For this review, take the finished solid that the model builds, in its own axes (mm). Give positions to 0.01 mm unless a question says otherwise; leave off trailing zeros. Loops run counter-clockwise (first coordinate to the right, second up) from the corner with the lowest first, then second, coordinate; pieces in that order, holes last.
```python
from build123d import *

# Parameters (mm, degrees)
SKETCH1_W                 = 220
SKETCH1_H                 = 220
BOSS_EXTRUDE1_DEPTH       = 6
SKETCH2_R                 = 6
CUT_EXTRUDE1_DEPTH        = 51
FILLET1_R                 = 10
F_4_0MM_DOWEL_HOLE1_D     = 4
F_4_0MM_DOWEL_HOLE1_DEPTH = 25.4
F_4_0MM_DOWEL_HOLE1_TIP   = 1.201721238


with BuildPart() as part:
    # Sketch1 → Boss-Extrude1 (new body)
    with BuildSketch(Plane(origin=(0, 0, 0), x_dir=(1, 0, 0), z_dir=(0, 1, 0))):
        Rectangle(SKETCH1_W, SKETCH1_H)
    extrude(amount=BOSS_EXTRUDE1_DEPTH)

    # Sketch2 → Cut-Extrude1 (cut)
    with BuildSketch(Plane(origin=(0, 6, 0), x_dir=(1, 0, 0), z_dir=(0, 1, 0))):
        with Locations(Location((0, 0, 0), (0, 0, 270))):
            Circle(SKETCH2_R)
    extrude(amount=-CUT_EXTRUDE1_DEPTH, mode=Mode.SUBTRACT)

    # Fillet1
    fillet1_edges = [part.edges().sort_by_distance(p)[0] for p in [
        (-110, 3, -110),
        (110, 3, -110),
        (110, 3, 110),
        (-110, 3, 110),
    ]]
    fillet(fillet1_edges, radius=FILLET1_R)

    # Ø4.0mm Dowel Hole1
    with Locations(Plane(origin=(0, 6, 0), x_dir=(1, 0, 0), z_dir=(0, 1, 0))):
        with Locations((-9.557884959, -94.152737777), (9.557884959, -94.152737777), (94.152737777, -9.557884959), (94.152737777, 9.557884959), (9.557884959, 94.152737777), (-9.557884959, 94.152737777), (-94.152737777, 9.557884959), (-94.152737777, -9.557884959)):
            Hole(F_4_0MM_DOWEL_HOLE1_D / 2, depth=F_4_0MM_DOWEL_HOLE1_DEPTH)
            with Locations((0, 0, -(F_4_0MM_DOWEL_HOLE1_DEPTH + F_4_0MM_DOWEL_HOLE1_TIP / 2))):  # 118° drill point
                Cone(0, F_4_0MM_DOWEL_HOLE1_D / 2, F_4_0MM_DOWEL_HOLE1_TIP, mode=Mode.SUBTRACT)


solid = part.part
```
Item 1: Take a section at B-B on z = 0. Give the boundary of the cut face in (x, y), and give its area (3 significant figures).
Answer:
outline: (-110, 0) - (-6, 0) - (-6, 6) - (-110, 6) - close; (6, 0) - (110, 0) - (110, 6) - (6, 6) - close
area: 1,250 mm2
Item 2: Take a section at A-A on x = 0. Give the boundary of the cut face in (y, z), and give its area (3 significant figures).
Answer:
outline: (0, -110) - (6, -110) - (6, -6) - (0, -6) - close; (0, 6) - (6, 6) - (6, 110) - (0, 110) - close
area: 1,250 mm2
Item 3: The part is to be moulded in two halves that separate along Z. For faces 1 (the flat face through (-1, 3, -110)), 2 (the cylindrical face through (-107.15, 3.04, 106.99)), 3 (the flat face through (-110, 3, 1)), 4 (the cylindrical face through (1.802, 3.042, 5.723)), say which applies: released by +Z, released by -Z, zero draft, split by the parting line, or undercut.
Answer:
face 1: released by -Z
face 2: released by +Z
face 3: zero draft
face 4: undercut
Item 4: Clearance check with a flat-ended pin moving along its axis: pin 1 Ø2.5 at (x, z) = (9.56, -94.15) entering from -Y. State where the tip first meets the part, or that it passes through.
Answer:
pin 1: passes through
